Print and shaded views of the part. All mm, measured from the part's lowest x, y and z. A direction names the side the tool comes from. Coordinates: 2 decimals unless noted, no trailing zeros. Order: outer loops, then holes, each group sorted by start corner. A loop starts at its lowest first (then second) coordinate and runs counter-clockwise, first axis right, second up. Notation, with made-up numbers: M 65,-38.5 L 115,-38.5 A18 ccw 115,-26.5 Z; hole C 45,-21 d7. An arc over 180 degrees is marked long. One line per item, written item: value.
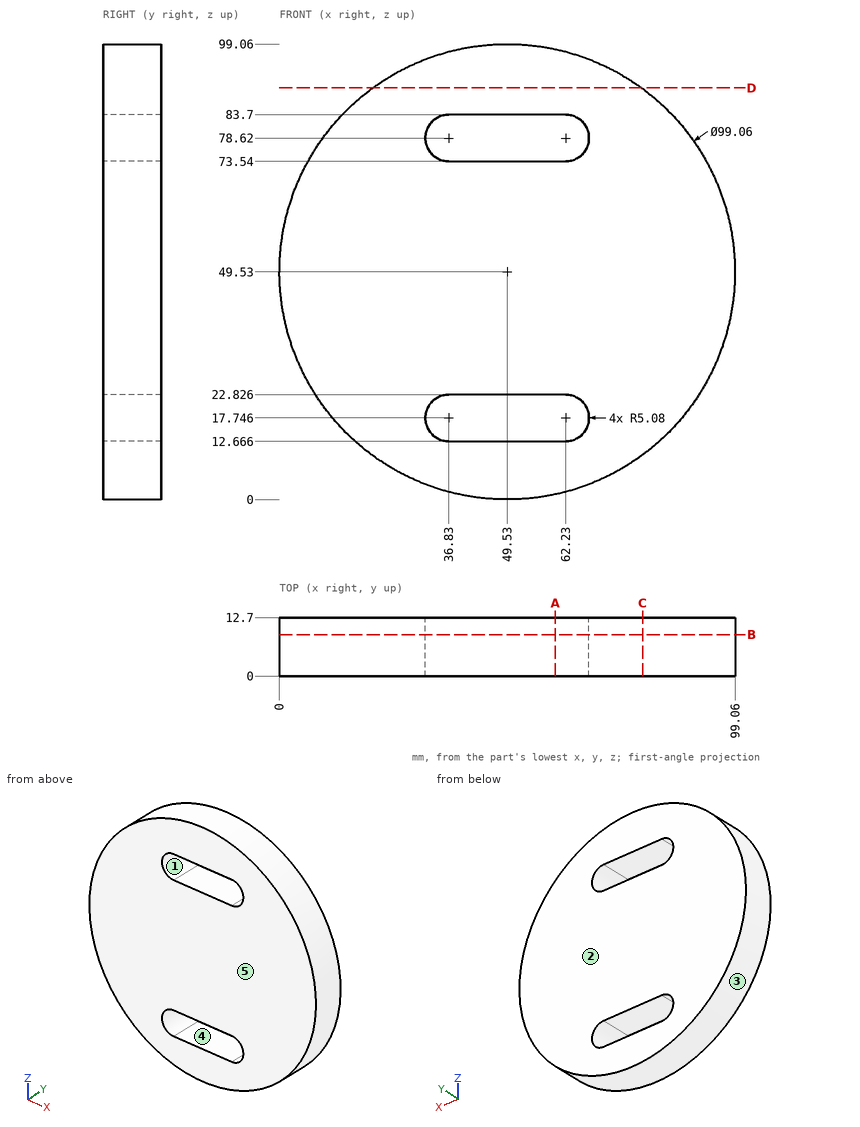
Q1. Which spindle directions (+Z, -Z, +X, -X, +Y, -Y) get a long thin tool onto all of the face, cutting with end or side? Do the marked faces 1 and 2. Say none if no direction does.
Recorded:
face 1: +Y, -Y
face 2: +Z, -Z, +X, -X, +Y
Q2. Mould opens along X. For the marked faces 3, 4 and 5 say: released by +X, released by -X, zero draft, split by the parting line, or undercut.
Recorded:
face 3: split by the parting line
face 4: undercut
face 5: zero draft
Q3. Pin check, flat tips, straight feed: pin 1 Ø1.5 at (x, y) = (51.5, 5.5) entering from -Z (3 decimals); pin 2 Ø4 at (x, y) = (45.5, 7) entering from +Z; pin 3 Ø3 at (y, z) = (4.5, 25) entering from +X. Stop position of each tip, or through.
Recorded:
pin 1: stops at z = 0.015
pin 2: stops at z = 99.02
pin 3: stops at x = 93.38
Q4. Slice it at A-A (x = 60). List the corners of the cut face in (y, z).
Recorded:
outline: M 0,1.12 L 12.7,1.12 L 12.7,12.67 L 0,12.67 Z; M 0,22.83 L 12.7,22.83 L 12.7,73.54 L 0,73.54 Z; M 0,83.7 L 12.7,83.7 L 12.7,97.94 L 0,97.94 Z
Q5. Slice it at B-B (y = 9). List the corners of the cut face in (x, z), plus the area to 3 significant figures.
Recorded:
outline: C 49.53,49.53 d99.06; hole M 36.83,12.67 L 62.23,12.67 A5.08 ccw 62.23,22.83 L 36.83,22.83 A5.08 ccw Z; hole M 36.83,73.54 L 62.23,73.54 A5.08 ccw 62.23,83.7 L 36.83,83.7 A5.08 ccw Z
area: 7,030 mm^2
Q6. Slice it at D-D (z = 89.5). List the corners of the cut face in (x, y).
Recorded:
outline: M 20.28,0 L 78.78,0 L 78.78,12.7 L 20.28,12.7 Z
Q7. Slice it at C-C (x = 79). List the corners of the cut face in (y, z), plus the area to 3 significant figures.
Recorded:
outline: M 0,9.72 L 12.7,9.72 L 12.7,89.34 L 0,89.34 Z
area: 1,010 mm^2
Q8. Drill centre lines: line 1 along Z through (x, y) = (66.5, 3.25); line 2 along Z through (x, y) = (55, 8.25); line 3 along X through (y, z) = (8.75, 74.5) (1 decimal). Where is each one in solid material? Low to high.
Recorded:
line 1: z = 3 to 14.99, 20.5 to 75.87, 81.37 to 96.06
line 2: z = 0.3 to 12.67, 22.83 to 73.54, 83.7 to 98.76
line 3: x = 6.8 to 33.9, 65.2 to 92.3
